```python
from build123d import *

# Parameters (mm, degrees)
PAD001_DEPTH        = 35
HOLE002_D           = 5.5
HOLE002_CSINK_D     = 10
HOLE002_CSINK_ANGLE = 90
SKETCH004_R         = 6.501169
SKETCH004_R_2       = 5.481256
POCKET_DEPTH        = 12.8390795694
SKETCH007_W         = 3.5
SKETCH007_H         = 35
POCKET002_DEPTH     = 1
CHAMFER_SIZE        = 0.99
FILLET007_R         = 3
FILLET008_R         = 1


with BuildPart() as part:
    # Sketch002 → Pad001 (new body)
    with BuildSketch(Plane.YZ):
        with BuildLine():
            Line((-191.8299400553, 608.417587482), (-180.7534222613, 635.3096898309))
            Line((-172.4316788603, 631.8820686779), (-180.7534222613, 635.3096898309))
            Line((-171.5440233176, 599.0713301394), (-172.4316788603, 631.8820686779))
            Line((-175.3524912653, 589.8249485827), (-171.5440233176, 599.0713301394))
            Line((-193.8452543786, 597.4418844782), (-175.3524912653, 589.8249485827))
            ThreePointArc((-193.8452543786, 597.4418844782), (-189.1063549521, 602.2446203225), (-191.8299400553, 608.417587482))
        make_face()
    extrude(amount=PAD001_DEPTH)

    # Hole002 (through all)
    with Locations(Plane(origin=(0, -366.2373103971, 150.8485291635), x_dir=(0, 0.3808467948, 0.9246381557), z_dir=(0, 0.9246381557, -0.3808467948))):
        with Locations((-506.967621, 13.13074), (501.5922183693, 17.5)):
            CounterSinkHole(HOLE002_D / 2, HOLE002_CSINK_D / 2, counter_sink_angle=HOLE002_CSINK_ANGLE)

    # Sketch004 (on DatumPlane) → Pocket (cut, through all)
    with BuildSketch(Plane(origin=(0, -366.2373103971, 150.8485291635), x_dir=(0, 0.3808467948, 0.9246381557), z_dir=(0, 0.9246381557, -0.3808467948))):
        with Locations((-506.967621, 13.13074)):
            Circle(SKETCH004_R)
        with Locations((501.5922183693, 17.5)):
            Circle(SKETCH004_R_2)
    extrude(amount=POCKET_DEPTH, mode=Mode.SUBTRACT)

    # Sketch007 (on Face6 of Pocket) → Pocket002 (cut)
    with BuildSketch(Plane(origin=(0, -378.2576064208, 155.7995374955), x_dir=(0, -0.3808467948, -0.9246381557), z_dir=(0, -0.9246381557, 0.3808467948))):
        with Locations((-513.5922183693, 17.5)):
            Rectangle(SKETCH007_W, SKETCH007_H)
    extrude(amount=-POCKET002_DEPTH, mode=Mode.SUBTRACT)

    # Chamfer
    chamfer_edges = [part.edges().sort_by_distance(p)[0] for p in [
        (17.5, -181.066536, 631.923769),
        (17.5, -182.3995, 628.687535),
    ]]
    chamfer(chamfer_edges, length=CHAMFER_SIZE)

    # Fillet007
    fillet007_edges = [part.edges().sort_by_distance(p)[0] for p in [
        (17.5, -175.352491, 589.824949),
        (17.5, -191.82994, 608.417587),
        (17.5, -171.544023, 599.07133),
        (17.5, -172.431679, 631.882069),
        (17.5, -180.753422, 635.30969),
    ]]
    fillet(fillet007_edges, radius=FILLET007_R)

    # Fillet008
    fillet008_edges = [part.edges().sort_by_distance(p)[0] for p in [
        (17.5, -193.845254, 597.441884),
    ]]
    fillet(fillet008_edges, radius=FILLET008_R)


solid = part.part
```
CAD build for the part. Positions are in the model's coordinates, mm. A direction names the side the tool comes from. Coordinates: 2 decimals unless noted, no trailing zeros. Write each loop counter-clockwise with the first axis right and the second up, starting at its lowest first coordinate (ties: lowest second). Pieces come first, ordered by that corner, then holes. Notation, with made-up numbers: (1.5, 47) -> (59.5, 47) arc R28 ccw to (59.5, 83) -> close; hole circle Ø3 at (-27.75, 41). An arc over 180 degrees is marked (long way). Return JSON: item names as keys, results as strings. Group by question number.
Q1. Cut at D-D, the plane z = 631.5. Give the cut face in (x, y).
Q2. Pull direction X, two halves, no side cores. Call faces 3 (the face through (17.74, -180.31, 634.15)), 4 (the face through (17.741, -175.146, 608.692)), 5 (the face through (0, -179, 613)): released by +X, released by -X, zero draft, split by the parting line, or undercut.
Q3. Cut at A-A, the plane y = -190. Give the cut face in (x, z).
Q4. Drill centre lines: line 1 (X direction, y = -176, z = 613.5); line 2 (Z direction, x = 19.5, y = -174.25); line 3 (Z direction, x = 22.5, y = -176.5). Where is each one in solid material? Low to high.
Q5. Cut at C-C, the plane z = 624. Give the cut face in (x, y).
Q6. Which spindle directions (+Z, -Z, +X, -X, +Y, -Y) get a long thin tool onto all of the face, cutting with end or side? Do faces 1 (the face through (17.745, -181.729, 630.315)), 2 (the face through (21.144, -187.222, 619.605)). Say none if no direction does.
Q7. Flat gauge pins, fed straight in: pin 1 (1.5 mm diameter, centred on y = -185.5, z = 627.5, fed in from +X); pin 2 (4 mm diameter, centred on y = -180, z = 617.5, fed in from -X); pin 3 (5 mm diameter, centred on x = 14.5, z = 629.5, fed in from -Y); pin 4 (1.5 mm diameter, centred on x = 22, y = -186, fed in from +Z). Where does each tip first touch, or does it go through?
Returned:
{
 "1": {"outline": "(0, -181.65) -> (35, -181.65) -> (35, -172.87) -> (0, -172.87) -> close"},
 "2": {"face 3": "zero draft", "face 4": "undercut", "face 5": "released by -X"},
 "3": {"outline": "(0, 595.86) -> (35, 595.86) -> (35, 600.02) -> (0, 600.02) -> close; (0, 606.63) -> (35, 606.63) -> (35, 612.86) -> (0, 612.86) -> close"},
 "4": {"line 1": "x = 0 to 13, 22 to 35", "line 2": "z = 592.51 to 608.73, 618.5 to 632.63", "line 3": "z = 590.78 to 633.56"},
 "5": {"outline": "(0, -185.41) -> (35, -185.41) -> (35, -172.22) -> (0, -172.22) -> close"},
 "6": {"face 1": "+X, -X, -Y", "face 2": "+Z, +X, -X, -Y"},
 "7": {"pin 1": "passes through", "pin 2": "stops at x = 0", "pin 3": "stops at y = -184.18", "pin 4": "stops at z = 624.39"}
}
